Autodesk Inventor part; units mm, degrees
ref_plane "YZ Plane" through (0, 0, 0) normal (1, 0, 0) x (0, 1, 0)
ref_plane "XZ Plane" through (0, 0, 0) normal (0, 1, 0) x (-1, 0, 0)
ref_plane "XY Plane" through (0, 0, 0) normal (0, 0, 1) x (1, 0, 0)
sketch "Náčrt1" plane through (0, 0, 0) normal (0, 0, 1) x (1, 0, 0)
  circle A0 centre (0, 0) radius 12.0945
  line L0 (0, 0) -> (0.5842, 13.9377)
  arc A1 (5.5661, 10.7376) -> (5.8875, 13.3827) centre (0.5319, 12.6914) ccw
  arc A2 (8.1555, 8.9311) -> (9.1506, 11.4029) centre (3.7986, 12.1212) ccw
  arc A3 (10.1892, 6.516) -> (11.7901, 8.646) centre (6.8063, 10.7251) ccw
  arc A4 (11.5284, 3.6568) -> (13.6261, 5.2999) centre (9.3503, 8.598) ccw
  arc A5 (12.0821, 0.5484) -> (14.5335, 1.5926) centre (11.257, 5.885) ccw
  arc A6 (11.8123, -2.5973) -> (14.4505, -2.2232) centre (12.3966, 2.771) ccw
  arc A7 (10.7376, -5.5661) -> (13.3827, -5.8875) centre (12.6914, -0.5319) ccw
  arc A8 (8.9311, -8.1555) -> (11.4029, -9.1506) centre (12.1212, -3.7986) ccw
  arc A9 (6.516, -10.1892) -> (8.646, -11.7901) centre (10.7251, -6.8063) ccw
  arc A10 (3.6568, -11.5284) -> (5.2999, -13.6261) centre (8.598, -9.3503) ccw
  arc A11 (0.5484, -12.0821) -> (1.5926, -14.5335) centre (5.885, -11.257) ccw
  line L1 (0, 0) -> (0, 15.3936)
  arc A12 (5.2999, 13.6261) -> (3.6568, 11.5284) centre (8.598, 9.3503) ccw
  arc A13 (8.646, 11.7901) -> (6.516, 10.1892) centre (10.7251, 6.8063) ccw
  arc A14 (11.4029, 9.1506) -> (8.9311, 8.1555) centre (12.1212, 3.7986) ccw
  arc A15 (13.3827, 5.8875) -> (10.7376, 5.5661) centre (12.6914, 0.5319) ccw
  arc A16 (14.4505, 2.2232) -> (11.8123, 2.5973) centre (12.3966, -2.771) ccw
  arc A17 (14.5335, -1.5926) -> (12.0821, -0.5484) centre (11.257, -5.885) ccw
  arc A18 (13.6261, -5.2999) -> (11.5284, -3.6568) centre (9.3503, -8.598) ccw
  arc A19 (11.7901, -8.646) -> (10.1892, -6.516) centre (6.8063, -10.7251) ccw
  arc A20 (9.1506, -11.4029) -> (8.1555, -8.9311) centre (3.7986, -12.1212) ccw
  arc A21 (5.8875, -13.3827) -> (5.5661, -10.7376) centre (0.5319, -12.6914) ccw
  arc A22 (2.2232, -14.4505) -> (2.5973, -11.8123) centre (-2.771, -12.3966) ccw
  arc A23 (5.8875, 13.3827) -> (5.2999, 13.6261) centre (0, 0) ccw
  arc A24 (9.1506, 11.4029) -> (8.646, 11.7901) centre (0, 0) ccw
  arc A25 (11.7901, 8.646) -> (11.4029, 9.1506) centre (0, 0) ccw
  arc A26 (13.6261, 5.2999) -> (13.3827, 5.8875) centre (0, 0) ccw
  arc A27 (14.5335, 1.5926) -> (14.4505, 2.2232) centre (0, 0) ccw
  arc A28 (14.4505, -2.2232) -> (14.5335, -1.5926) centre (0, 0) ccw
  arc A29 (13.3827, -5.8875) -> (13.6261, -5.2999) centre (0, 0) ccw
  arc A30 (11.4029, -9.1506) -> (11.7901, -8.646) centre (0, 0) ccw
  arc A31 (8.646, -11.7901) -> (9.1506, -11.4029) centre (0, 0) ccw
  arc A32 (1.5926, -14.5335) -> (2.2232, -14.4505) centre (0, 0) ccw
  arc A33 (5.2999, -13.6261) -> (5.8875, -13.3827) centre (0, 0) ccw
  dimension "d0" = 24.189
  dimension "d13" = 150
  dimension "d19" = 150
sketch "Náčrt2" plane through (0, 0, 0) normal (0, 0, 1) x (1, 0, 0)
  circle A0 centre (0, 0) radius 12.0945
  circle A1 centre (0, 0) radius 12.0945
extrude "Vysunutí1" add sketch "Náčrt2" along normal blind 4
extrude "Vysunutí2" add sketch "Náčrt1" along normal blind 4 contours A0 A12 A23 A1
pattern_circular "Kruhové pole1" count 11 over 150 about axis through (0, 0, 0) along (0, 0, -1) of "Vysunutí2"
sketch "Náčrt3" plane through (0, 0, 4) normal (0, 0, 1) x (1, 0, 0)
  line L0 (0, 0) -> (-4.0046, 30.5002)
  circle A0 centre (-4.0046, 30.5002) radius 1.825
  arc A1 (-0.0386, 31.0209) -> (-7.9706, 29.9795) centre (-4.0046, 30.5002) ccw
  line L1 (-3.966, -0.5207) -> (-7.9706, 29.9795)
  line L2 (3.966, 0.5207) -> (-0.0386, 31.0209)
  line L3 (-5.0618, 7.8256) -> (2.8701, 8.867)
  dimension "d29" = 30.762
  dimension "d30" = 3.65
  dimension "d31" = 8
  dimension "d32" = 4
  dimension "d33" = 4
extrude "Vysunutí3" add sketch "Náčrt3" against normal blind 4
sketch "Náčrt4" plane through (0, 0, 4) normal (0, 0, 1) x (1, 0, 0)
  circle A0 centre (0, 0) radius 2.4
  line L0 (0, 0) -> (0, -4.4)
  circle A1 centre (0, -4.4) radius 1.3
  line L1 (0, 0) -> (0, 4.4)
  circle A2 centre (0, 4.4) radius 1.3
  dimension "d36" = 4.8
  dimension "d37" = 4.4
  dimension "d38" = 2.6
  dimension "d39" = 4.4
  dimension "d40" = 2.6
extrude "Vysunutí4" cut sketch "Náčrt4" against normal blind 4
properties part number "zubate_kolo2" material "ABS Plastic"
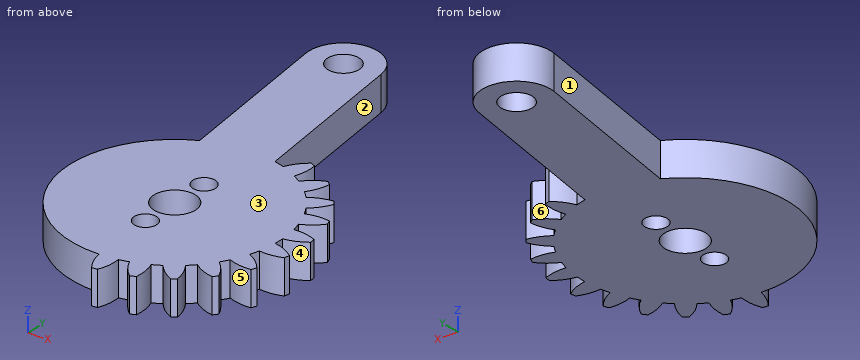
CAD build for the part. Positions are in the model's coordinates, mm. Face numbers are marked on the shaded views. A direction names the side the tool comes from. Round coordinates to 2 decimals unless told otherwise and drop trailing zeros. Order: outer loops, then holes, each group sorted by start corner. A loop starts at its lowest first (then second) coordinate and runs counter-clockwise, first axis right, second up.
Q1. Slice it at A-A (y = 0). Write the cut outline in (x, z), and give its area (3 significant figures).
Q2. Which spindle directions (+Z, -Z, +X, -X, +Y, -Y) get a long thin tool onto all of the face, cutting with end or side? Do the marked faces 4, 5 and 6. Say none if no direction does.
Q3. Two-plate mould, pull along Y, no slides. Class the marked faces 1, 2 and 3: pulls with the +Y half, pulls with the -Y half, needs draft (parallel to the pull), parting line crosses it, or undercut.
Q4. Drop flat-ended pins along their axis: pin 1 (1.5 mm diameter, centred on x = -5, z = 2.5, fed in from +Y); pin 2 (1.5 mm diameter, centred on x = 0.5, z = 2, fed in from -Y); pin 3 (1.5 mm diameter, centred on x = 0, z = 2.5, fed in from +Y). Give the stop position or say it passes through.
Q5. Slice it at D-D (x = -9.5). Write the cut outline in (y, z), and give its area (3 significant figures).
Q6. Slice it at C-C (z = 2.9). State how many separate pieces and enclosed holes the cut face has, and give its area (3 significant figures).
Q7. Slice it at B-B (x = -4.25). Write the cut outline in (y, z), and give its area (3 significant figures).
Q8. Wall check: L1, parallel to Y at x = -4, z = 1.3; L2, parallel to Y at x = 12.5, z = 2.6; L3, parallel to Y at x = 12.75, z = 2.35. Give the ranges that are in metal, low to high.
Results below:
1. outline: (-12.09, 0) - (-2.4, 0) - (-2.4, 4) - (-12.09, 4) - close; (2.4, 0) - (12.09, 0) - (12.09, 4) - (2.4, 4) - close
1. area: 77.6 mm2
2. face 4: +Z, -Z, +X
2. face 5: +Z, -Z
2. face 6: +Z, -Z, +Y
3. face 1: undercut
3. face 2: pulls with the +Y half
3. face 3: needs draft
4. pin 1: stops at y = 34.49
4. pin 2: stops at y = -14.03
4. pin 3: stops at y = 32.83
5. outline: (-7.49, 0) - (7.49, 0) - (7.49, 4) - (-7.49, 4) - close
5. area: 59.9 mm2
6. separate pieces: 1
6. enclosed holes: 4
6. area: 641 mm2
7. outline: (-11.32, 0) - (28.69, 0) - (28.69, 4) - (-11.32, 4) - close; (32.31, 0) - (34.49, 0) - (34.49, 4) - (32.31, 4) - close
7. area: 169 mm2
8. L1: y = -11.41 to 28.68, 32.33 to 34.5
8. L2: y = -5.93 to -4.21, -2.63 to -0.63, 0.63 to 2.63, 4.21 to 5.93
8. L3: y = -5.93 to -4.4, -2.62 to -0.7, 0.7 to 2.62, 4.4 to 5.93
